Verification items for the finished model (mm, model axes). Coordinates: 2 decimals unless noted, no trailing zeros. Write item = value, one per line. Start each with the question number.
(1) Section check A-A (z = 1.75). State how many separate pieces and enclosed holes the cut face has, plus the area to 3 significant figures.
(2) Material ranges on probe 1 along Y at (x, z) = (0, 3.75); probe 2 along Y at (x, z) = (27.5, 1.5); probe 3 along X at (y, z) = (-27, 6.25), recorded low to high. Write a range as [from, to].
(3) Gauge pin test, flat ends, axial feed: pin 1 Ø6 at (x, z) = (-27, 2) entering from -Y; pin 2 Ø1 at (y, z) = (10.5, 5) entering from +X; pin 3 Ø5 at (x, z) = (3.5, 3) entering from -Y; pin 4 Ø5 at (x, y) = (-13.462, 0) entering from +Z. Record the tip position at first contact, or that the pin passes through.
(4) Mould release check, pull along X, two halves, no side actions. Record for faces 1 (the face through (21.473, 24.062, 6.432)), 2 (the face through (0.516, 30.996, 6.268)), 3 (the face through (-1, 1, 12.7)): released by +X, released by -X, zero draft, split by the parting line, or undercut.
```python
from build123d import *

# Parameters (mm, degrees)
SKETCH1_R          = 44.45
EXTRUDE1_DEPTH     = 12.7
SKETCH2_R          = 3.9624
CUT_EXTRUDE3_DEPTH = 13.7
SKETCH3_R          = 3.9624
CUT_EXTRUDE4_DEPTH = 13.7
CIRPATTERN1_COUNT  = 4
CHAMFER1_SIZE      = 0.508
SKETCH4_R          = 3.9624
CUT_EXTRUDE8_DEPTH = 13.7
CIRPATTERN3_COUNT  = 4
CHAMFER2_SIZE      = 0.508
CHAMFER3_SIZE      = 0.508


with BuildPart() as part:
    # Sketch1 → Extrude1 (new body)
    with BuildSketch(Plane.XY):
        Circle(SKETCH1_R)
    extrude(amount=EXTRUDE1_DEPTH)

    # Sketch2 → Cut-Extrude3 (cut, through all)
    with BuildSketch(Plane.XY):
        with Locations((0, 13.462)):
            Circle(SKETCH2_R)
        with Locations((13.462, 0)):
            Circle(SKETCH2_R)
        with Locations((0, -13.462)):
            Circle(SKETCH2_R)
        with Locations((-13.462, 0)):
            Circle(SKETCH2_R)
    extrude(amount=CUT_EXTRUDE3_DEPTH, mode=Mode.SUBTRACT)

    # Sketch3 → Cut-Extrude4 (cut, through all)
    with BuildSketch(Plane.XY):
        with Locations((0, -34.925)):
            Circle(SKETCH3_R)
    cut_extrude4 = extrude(amount=CUT_EXTRUDE4_DEPTH, mode=Mode.SUBTRACT)

    # CirPattern1: Cut-Extrude4 ×4 about axis
    cirpattern1_axis = Axis((0, 0, 0), (0, 0, 1))
    for i in range(1, CIRPATTERN1_COUNT):
        add(cut_extrude4.rotate(cirpattern1_axis, i * 360 / CIRPATTERN1_COUNT), mode=Mode.SUBTRACT)

    # Chamfer1
    chamfer1_edges = [part.edges().sort_by_distance(p)[0] for p in [
        (-3.9624, 13.462, 0),
        (-3.9624, 13.462, 12.7),
        (9.4996, 0, 12.7),
        (-3.9624, -13.462, 12.7),
        (-3.9624, -34.925, 0),
        (-3.9624, -34.925, 12.7),
        (34.925, -3.9624, 0),
        (34.925, -3.9624, 12.7),
        (3.9624, 34.925, 0),
        (3.9624, 34.925, 12.7),
        (-34.925, 3.9624, 0),
        (-34.925, 3.9624, 12.7),
        (-17.4244, 0, 12.7),
    ]]
    chamfer(chamfer1_edges, length=CHAMFER1_SIZE)

    # Sketch4 → Cut-Extrude8 (cut, through all)
    with BuildSketch(Plane.XY.offset(12.7)):
        with Locations((-25.252480212, -25.252480212)):
            Circle(SKETCH4_R)
    cut_extrude8 = extrude(amount=-CUT_EXTRUDE8_DEPTH, mode=Mode.SUBTRACT)

    # CirPattern3: Cut-Extrude8 ×4 about axis
    cirpattern3_axis = Axis((0, 0, 0), (0, 0, 1))
    for i in range(1, CIRPATTERN3_COUNT):
        add(cut_extrude8.rotate(cirpattern3_axis, i * 360 / CIRPATTERN3_COUNT), mode=Mode.SUBTRACT)

    # Chamfer2
    chamfer2_edges = [part.edges().sort_by_distance(p)[0] for p in [
        (9.4996, 0, 0),
        (-3.9624, -13.462, 0),
        (-17.4244, 0, 0),
        (-29.214880212, -25.252480212, 0),
        (-29.214880212, -25.252480212, 12.7),
        (25.252480212, -29.214880212, 0),
        (25.252480212, -29.214880212, 12.7),
        (29.214880212, 25.252480212, 0),
        (29.214880212, 25.252480212, 12.7),
        (-25.252480212, 29.214880212, 0),
        (-25.252480212, 29.214880212, 12.7),
    ]]
    chamfer(chamfer2_edges, length=CHAMFER2_SIZE)

    # Chamfer3
    chamfer3_edges = [part.edges().sort_by_distance(p)[0] for p in [
        (-44.45, 0, 0),
        (-44.45, 0, 12.7),
    ]]
    chamfer(chamfer3_edges, length=CHAMFER3_SIZE)


solid = part.part
```
Response:
q1.separate_pieces = 1
q1.enclosed_holes = 12
q1.area = 5,620 mm2
q2.probe_1 = [-44.45, -38.89], [-30.96, -17.42], [-9.5, 9.5], [17.42, 30.96], [38.89, 44.45]
q2.probe_2 = [-34.92, -28.52], [-21.99, 21.99], [28.52, 34.92]
q2.probe_3 = [-35.31, -28.81], [-21.7, 21.7], [28.81, 35.31]
q3.pin_1 = -37.41
q3.pin_2 = 43.31
q3.pin_3 = -44.44
q3.pin_4 = through
q4.face_1 = undercut
q4.face_2 = undercut
q4.face_3 = zero draft
